Verification items for this drawing (mm, ordinates from the low corner). Round coordinates to 2 decimals unless told otherwise and drop trailing zeros. Write each loop counter-clockwise with the first axis right and the second up, starting at its lowest first coordinate (ties: lowest second). Pieces come first, ordered by that corner, then holes. Notation, with made-up numbers: M 57,5 L 66,5 A34 ccw 66,39 Z; hole C 21.5,-29.5 d2. An arc over 180 degrees is marked long. One line per question, with ' | ' between items. Start each with the question number.
Q1. Release check for a two-part mould opening along Y. For the marked faces 1, 2 and 3 record: released by +Y, released by -Y, zero draft, split by the parting line, or undercut.
Q2. Gauge pin test, flat ends, axial feed: pin 1 (3 mm diameter, centred on y = 89, z = 25.5, fed in from -X); pin 2 (4 mm diameter, centred on y = 62.5, z = 6, fed in from +X); pin 3 (22 mm diameter, centred on x = 60.5, y = 14.5, fed in from +Z). Record the tip position at first contact, or that the pin passes through.
Q3. Cross-section at B-B (z = 8.5). Record the boundary of the cut face in (x, y), then the cut area to 3 significant figures.
Q4. Thickness scan on line 1 along Y through (x, z) = (86, 19.25); line 2 along X through (y, z) = (73.5, 4.5); line 3 along Z through (x, y) = (51.5, 10). Record the ranges inside material, lowest first. Write a range as from..to.
Q5. Cross-section at C-C (y = 70). Record the boundary of the cut face in (x, z).
Q6. Cross-section at A-A (x = 396.5). Record the boundary of the cut face in (y, z).
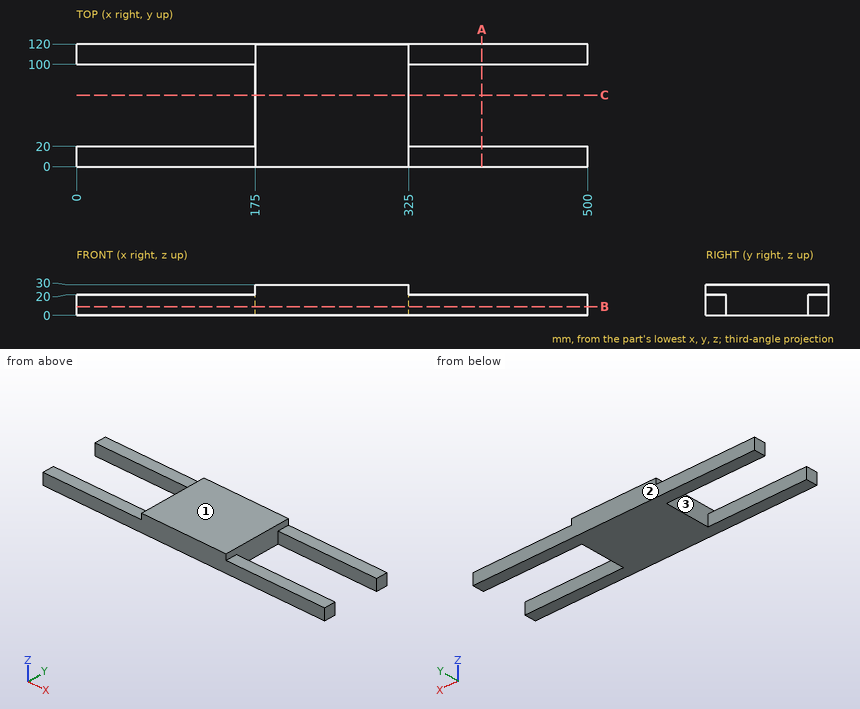
Determined:
1) face 1: zero draft | face 2: released by +Y | face 3: undercut
2) pin 1: stops at x = 175 | pin 2: stops at x = 325 | pin 3: stops at z = 20
3) outline: M 0,0 L 500,0 L 500,20 L 325,20 L 325,100 L 500,100 L 500,120 L 0,120 L 0,100 L 175,100 L 175,20 L 0,20 Z | area: 32,000 mm²
4) line 1: y = 0..20, 100..120 | line 2: x = 175..325 | line 3: z = 0..20
5) outline: M 175,0 L 325,0 L 325,30 L 175,30 Z
6) outline: M 0,0 L 20,0 L 20,20 L 0,20 Z; M 100,0 L 120,0 L 120,20 L 100,20 Z
